Part print with two shaded views. Sizes in mm from the minimum x, y, z corner. A direction names the side the tool comes from. Round coordinates to 2 decimals unless told otherwise and drop trailing zeros. Write each loop counter-clockwise with the first axis right and the second up, starting at its lowest first coordinate (ties: lowest second). Pieces come first, ordered by that corner, then holes. Notation, with made-up numbers: M -36.5,81.5 L -25.5,81.5 A19 cw -25.5,106.5 Z; hole C 58.25,8 d8. An arc over 180 degrees is marked long. One line per question, with ' | ' between items. Start each with the question number.
1) Mould opens along Y. For the marked faces 1, 2 and 3 say: pulls with the +Y half, pulls with the -Y half, needs draft (parallel to the pull), parting line crosses it, or undercut.
2) Saw through at C-C (z = 0.3). List the corners of the cut face in (x, y) (1 decimal).
3) Tool access for the marked faces 4 and 5: list every direction of +Z, -Z, +X, -X, +Y, -Y with a clear straight run to the whole face (end or side of a thin tool).
4) Wall check: probe 1 along X at (y, z) = (11, 1.25); probe 2 along X at (y, z) = (14.75, 2); probe 3 along Y at (x, z) = (15, 0.35). Give the ranges that are in metal, low to high. Write a range as [from, to].
5) Saw through at B-B (y = 6.5). List the corners of the cut face in (x, z).
6) Saw through at A-A (x = 14.25). List the corners of the cut face in (y, z).
7) Drop flat-ended pins along their axis: pin 1 Ø1 at (x, z) = (13, 1.5) entering from -Y (1 decimal); pin 2 Ø0.9 at (y, z) = (12, 1) entering from -X; pin 3 Ø0.9 at (x, z) = (9.5, 2) entering from -Y. Give the stop position or say it passes through.
8) Saw through at D-D (x = 5.75). List the corners of the cut face in (y, z).
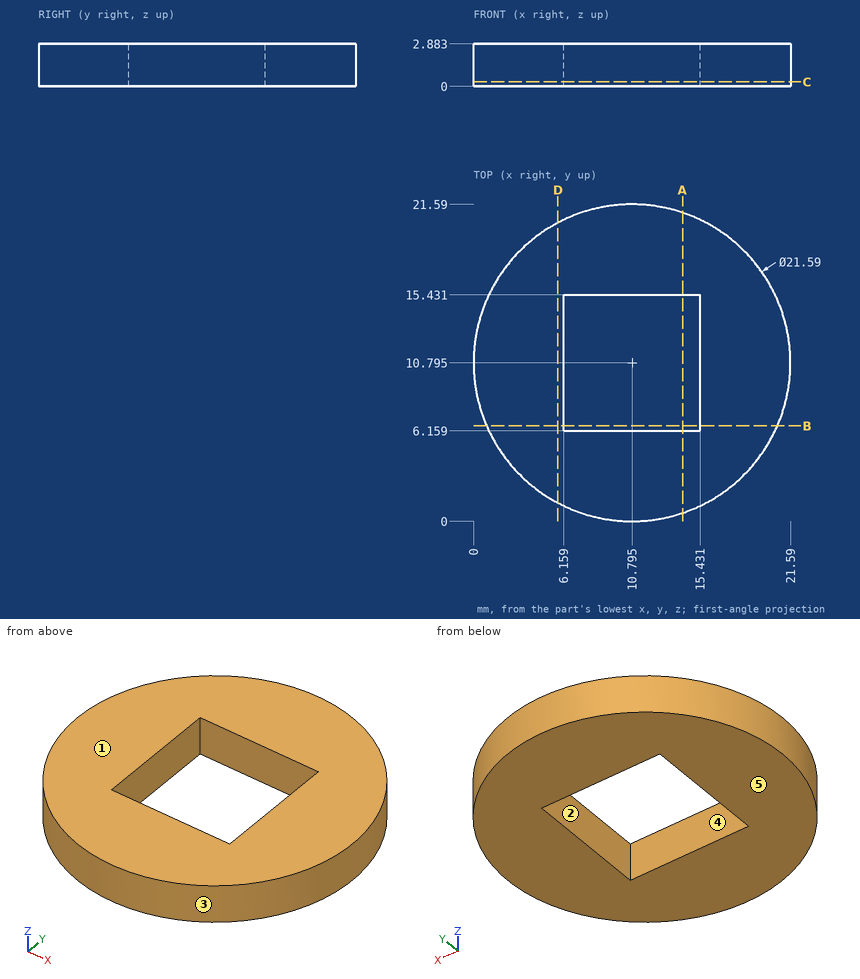
Answer key:
1) face 1: needs draft | face 2: undercut | face 3: parting line crosses it
2) outline: C 10.8,10.8 d21.6; hole M 6.2,6.2 L 15.4,6.2 L 15.4,15.4 L 6.2,15.4 Z
3) face 4: +Z, -Z | face 5: -Z, +X, -X, +Y, -Y
4) probe 1: x = [0, 6.16], [15.43, 21.59] | probe 2: x = [0.75, 6.16], [15.43, 20.84] | probe 3: y = [0.85, 6.16], [15.43, 20.74]
5) outline: M 0.89,0 L 6.16,0 L 6.16,2.88 L 0.89,2.88 Z; M 15.43,0 L 20.7,0 L 20.7,2.88 L 15.43,2.88 Z
6) outline: M 0.57,0 L 6.16,0 L 6.16,2.88 L 0.57,2.88 Z; M 15.43,0 L 21.02,0 L 21.02,2.88 L 15.43,2.88 Z
7) pin 1: stops at y = 0.1 | pin 2: stops at x = 0.03 | pin 3: stops at y = 0.03
8) outline: M 1.25,0 L 20.34,0 L 20.34,2.88 L 1.25,2.88 Z
